```python
from build123d import *

# Parameters (mm, degrees)
F0_R         = 25.4
F1_DEPTH     = 9.525
F2_R         = 6.35
F3_DEPTH     = 4.572
F4_R         = 25.4
F4_R_2       = 6.35
F5_DEPTH     = 9.525
F6_R         = 5.08
F7_R         = 10.9834381756
F8_DEPTH     = 2.54
F9_R         = 8.4850918215
F10_DEPTH    = 2.54
F11_R        = 6.7919077929
F12_DEPTH    = 2.54
F13_R        = 10.98296
F10_FACE_R   = 8.4850918215
F10_FACE_R_2 = 6.7919077929
F14_DEPTH    = 2.54
F15_R        = 8.4836
F16_DEPTH    = 2.54
F17_R        = 6.7945
F18_DEPTH    = 2.54


with BuildPart() as f1:
    # F0 (on Top) → F1 (new body)
    with BuildSketch(Plane.XY):
        Circle(F0_R)
    extrude(amount=F1_DEPTH)

    # F2 (on face) → F3 (join)
    with BuildSketch(Plane.XY.offset(9.525)):
        Circle(F2_R)
    extrude(amount=F3_DEPTH)

    # F0 (on Top) + F4 (on face) → F5 (join)
    with BuildSketch(Plane.XY):
        Circle(F0_R)
    with BuildSketch(Plane.XY.offset(14.097)):
        Circle(F4_R)
        Circle(F4_R_2, mode=Mode.SUBTRACT)
        Circle(F4_R_2)
    extrude(amount=F5_DEPTH)

    # F6
    f6_edges = [f1.edges().sort_by_distance(p)[0] for p in [
        (-25.4, 0, 23.622),
        (-25.4, 0, 0),
    ]]
    fillet(f6_edges, radius=F6_R)

    # F7 (on face) → F8 (join)
    with BuildSketch(Plane.XY.offset(23.622)):
        Circle(F7_R)
    extrude(amount=F8_DEPTH)

    # F9 (on face) → F10 (join)
    with BuildSketch(Plane.XY.offset(26.162)):
        Circle(F9_R)
    extrude(amount=F10_DEPTH)

    # F11 (on face) → F12 (join)
    with BuildSketch(Plane.XY.offset(28.702)):
        Circle(F11_R)
    extrude(amount=F12_DEPTH)

    # F13 (on face) + F10_face (on face) → F14 (join)
    with BuildSketch(Plane(origin=(0, 0, 0), x_dir=(1, 0, 0), z_dir=(0, 0, -1))):
        Circle(F13_R)
    with BuildSketch(Plane.XY.offset(28.702)):
        Circle(F10_FACE_R)
        Circle(F10_FACE_R_2, mode=Mode.SUBTRACT)
    extrude(amount=F14_DEPTH, dir=(0, 0, -1))

    # F15 (on face) → F16 (join)
    with BuildSketch(Plane(origin=(0, 0, -2.54), x_dir=(1, 0, 0), z_dir=(0, 0, -1))):
        Circle(F15_R)
    extrude(amount=F16_DEPTH)

    # F17 (on face) → F18 (join)
    with BuildSketch(Plane(origin=(0, 0, -5.08), x_dir=(1, 0, 0), z_dir=(0, 0, -1))):
        Circle(F17_R)
    extrude(amount=F18_DEPTH)


solid = f1.part
```
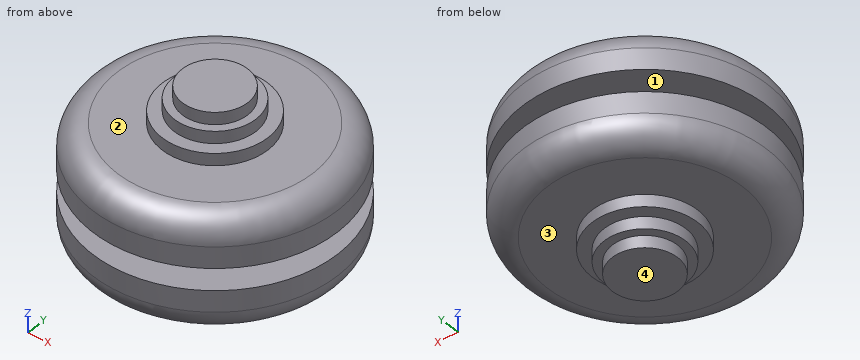
Geometry: final body of the model. Coordinates: model frame, mm. Face numbers are marked on the shaded views. A direction names the side the tool comes from. Round coordinates to 2 decimals unless told otherwise and drop trailing zeros. Write each loop counter-clockwise with the first axis right and the second up, starting at its lowest first coordinate (ties: lowest second). Pieces come first, ordered by that corner, then holes.
Item 1: Section query B-B (z = 25). Return loops of the section in (x, y), plus the area to 3 significant figures.
Item 2: Material intervals for L1, parallel to Z at x = 10.5, y = -11.5 (3 decimals); L2, parallel to Z at x = -4, y = -7 (3 decimals); L3, parallel to Y at x = 0, z = 24.5, sorted ascending.
Item 3: Pin query (flat end, axial travel): P1, Ø5, axis at x = -16, y = -17.5, coming from the +Z side; P2, Ø4, axis at x = 1.5, y = -12, coming from the -Z side; P3, Ø10, axis at x = 8, y = -10.5, coming from the +Z side; P4, Ø10, axis at y = 0.5, z = 5, coming from the -X side. Return the tip coordinate at first contact, or that it passes through.
Item 4: Set-up query: the marked faces 1, 2, 3 and 4. Return all of +Z, -Z, +X, -X, +Y, -Y with unobstructed straight access to the full face (end or side cutting, diameter ignored); none if empty.
Item 5: Section query A-A (z = 17). Return loops of the section in (x, y), plus the area to 3 significant figures.
Completed:
1. outline: circle Ø21.97 at (0, 0)
1. area: 379 mm2
2. L1: z = 0 to 9.525, 14.097 to 23.622
2. L2: z = -5.08 to 9.525, 14.097 to 28.702
2. L3: y = -10.98 to 10.98
3. P1: stops at z = 23.54
3. P2: stops at z = -2.54
3. P3: stops at z = 28.7
3. P4: stops at x = -25.4
4. face 1: none
4. face 2: +Z
4. face 3: -Z
4. face 4: -Z, +X, -X, +Y, -Y
5. outline: circle Ø50.8 at (0, 0)
5. area: 2,030 mm2
